Input: part model. Units: mm. Frame: model coordinates. A direction names the side the tool comes from. Round coordinates to 2 decimals unless told otherwise and drop trailing zeros. Loops run counter-clockwise (first coordinate to the right, second up) from the corner with the lowest first, then second, coordinate; pieces in that order, holes last. Notation, with made-up numbers: M -20.5,-31 L -1.5,-31 A15 ccw -1.5,-10 Z; hole C 5,43 d2. An arc over 180 degrees is marked long. Return JSON: item names as keys, results as strings. Group by question number.
1) Section C-C (y = 0). Output: boundary loops of the cut face in (x, z) (3 decimals), plus the area to 3 significant figures.
2) Mould query, pull axis Y, two halves, no side actions, for faces 1 (the face through (-11.59, -15.12, 11.05)), 2 (the face through (-8, -9, -15.875)), 3 (the face through (-61.99, -13.77, -0.22)). Classes: +Y half, -Y half, draft (parallel to the pull), parting line (faces both ways), or undercut.
3) Contact query for flat-ended pins moving along their axis: P1, Ø3.5, axis at y = 13, z = 5, coming from the -X side; P2, Ø1, axis at y = -13, z = -11, coming from the +X side; P3, Ø8, axis at x = -35.5, y = -3.5, coming from the +Z side. Output: stop coordinate, or through.
4) Material intervals for line 1 (X direction, y = 0, z = 13); line 2 (X direction, y = 0, z = 6); line 3 (Y direction, x = 8, z = -10.5), sorted ascending. Write a range as from..to.
5) Section B-B (x = 0). Output: boundary loops of the cut face in (y, z) (3 decimals), plus the area to 3 significant figures.
6) Access query for faces 4 (the face through (43, -29, -15.875)), 5 (the face through (-49.592, -11.012, -11.046)), 6 (the face through (-3.175, 13, 0)), 7 (the face through (43, 29, 15.875)), 8 (the face through (-49.592, -11.012, 11.179)). Directions: +Z, -Z, +X, -X, +Y, -Y. A direction counts if a zero-diameter tool reaches every point of the face in a straight line with its end or side. Return the directions, or none.
7) Section A-A (z = 11). Output: boundary loops of the cut face in (x, y) (3 decimals).
from build123d import *

# Parameters (mm, degrees)
SKETCH4_W          = 6.35
SKETCH4_H          = 3.175
CUT_EXTRUDE1_DEPTH = 32.75


with BuildPart() as part:
    # Sketch1 → Revolve1 (revolve)
    with BuildSketch(Plane(origin=(0, 0, 0), x_dir=(0, 0, -1), z_dir=(1, 0, 0))):
        Polygon((15.875, 11.509375), (-15.875, 11.509375), (-15.875, 19.05), (-6.35, 19.05), (-6.35, 50.8), (-15.875, 50.8), (-15.875, 63.5), (15.875, 63.5), (15.875, 50.8), (6.35, 50.8), (6.35, 19.05), (15.875, 19.05), align=None)
    revolve(axis=Axis((0, 0, 34.214514903), (0, 0, -1)))

    # Sketch4 → Cut-Extrude1 (cut, through all)
    with BuildSketch(Plane(origin=(0, 0, -15.875), x_dir=(-1, 0, 0), z_dir=(0, 0, -1))):
        with Locations((0, 12.650279393)):
            Rectangle(SKETCH4_W, SKETCH4_H)
    extrude(amount=-CUT_EXTRUDE1_DEPTH, mode=Mode.SUBTRACT)


solid = part.part
Returned:
{
 "1": {"outline": "M -63.5,-15.875 L -50.8,-15.875 L -50.8,-6.35 L -19.05,-6.35 L -19.05,-15.875 L -11.509,-15.875 L -11.509,15.875 L -19.05,15.875 L -19.05,6.35 L -50.8,6.35 L -50.8,15.875 L -63.5,15.875 Z; M 11.509,-15.875 L 19.05,-15.875 L 19.05,-6.35 L 50.8,-6.35 L 50.8,-15.875 L 63.5,-15.875 L 63.5,15.875 L 50.8,15.875 L 50.8,6.35 L 19.05,6.35 L 19.05,15.875 L 11.509,15.875 Z", "area": "2,090 mm^2"},
 "2": {"face 1": "undercut", "face 2": "draft", "face 3": "parting line"},
 "3": {"P1": "stops at x = -62.5", "P2": "stops at x = 62.26", "P3": "stops at z = 6.35"},
 "4": {"line 1": "x = -63.5..-50.8, -19.05..-11.51, 11.51..19.05, 50.8..63.5", "line 2": "x = -63.5..-11.51, 11.51..63.5", "line 3": "y = -62.99..-50.17, -17.29..-8.27, 8.27..17.29, 50.17..62.99"},
 "5": {"outline": "M -63.5,-15.875 L -50.8,-15.875 L -50.8,-6.35 L -19.05,-6.35 L -19.05,-15.875 L -11.509,-15.875 L -11.509,15.875 L -19.05,15.875 L -19.05,6.35 L -50.8,6.35 L -50.8,15.875 L -63.5,15.875 Z; M 14.238,-15.875 L 19.05,-15.875 L 19.05,-6.35 L 50.8,-6.35 L 50.8,-15.875 L 63.5,-15.875 L 63.5,15.875 L 50.8,15.875 L 50.8,6.35 L 19.05,6.35 L 19.05,15.875 L 14.238,15.875 Z", "area": "2,010 mm^2"},
 "6": {"face 4": "-Z, +X, -X, +Y, -Y", "face 5": "-Z", "face 6": "+Z, -Z", "face 7": "+Z, +X, -X, +Y, -Y", "face 8": "+Z"},
 "7": {"outline": "C 0,0 d127; C 0,0 d38.1; hole C 0,0 d101.6; hole M -3.175,11.063 A11.509 ccw long 3.175,11.063 L 3.175,14.238 L -3.175,14.238 Z"}
}
